Check sheet for the modelled part. Datum: model origin and axes. Units: mm. A direction names the side the tool comes from. Round coordinates to 2 decimals unless told otherwise and drop trailing zeros. One line per item, written item: value.
Autodesk Inventor part; units mm, degrees
ref_plane "YZ Plane" through (0, 0, 0) normal (1, 0, 0) x (0, 1, 0)
ref_plane "XZ Plane" through (0, 0, 0) normal (0, 1, 0) x (-1, 0, 0)
ref_plane "XY Plane" through (0, 0, 0) normal (0, 0, 1) x (1, 0, 0)
sketch "Sketch_1" plane through (0, 0, 0) normal (0, 0, 1) x (1, 0, 0)
  arc A0 (-7.5, 2) -> (-7.2, 1.7) centre (-7.2, 2) ccw
  line L0 (-7.2, 1.7) -> (-6.4, 1.7)
  line L1 (-6.4, 1.7) -> (-6.4, 2.85)
  line L2 (-6.4, 2.85) -> (-3.8, 2.85)
  line L3 (-3.8, 2.85) -> (-2.8, 1.85)
  line L4 (-2.8, 1.85) -> (-2.8, 0.5196)
  line L5 (-2.8, 0.5196) -> (-2.5, 0)
  line L6 (-2.5, 0) -> (-2.8, -0.5196)
  line L7 (-2.8, -0.5196) -> (-2.8, -1.85)
  line L8 (-2.8, -1.85) -> (-3.8, -2.85)
  line L9 (-3.8, -2.85) -> (-6.4, -2.85)
  line L10 (-6.4, -2.85) -> (-6.4, -1.7)
  line L11 (-6.4, -1.7) -> (-7.2, -1.7)
  arc A1 (-7.2, -1.7) -> (-7.5, -2) centre (-7.2, -2) ccw
  line L12 (-7.5, -2) -> (-7.5, -6.5)
  arc A2 (-7.5, -6.5) -> (-6.5, -7.5) centre (-6.5, -6.5) ccw
  line L13 (-6.5, -7.5) -> (-2, -7.5)
  arc A3 (-2, -7.5) -> (-1.7, -7.2) centre (-2, -7.2) ccw
  line L14 (-1.7, -7.2) -> (-1.7, -6.4)
  line L15 (-1.7, -6.4) -> (-2.85, -6.4)
  line L16 (-2.85, -6.4) -> (-2.85, -3.8)
  line L17 (-2.85, -3.8) -> (-1.85, -2.8)
  line L18 (-1.85, -2.8) -> (-0.5196, -2.8)
  line L19 (-0.5196, -2.8) -> (0, -2.5)
  line L20 (0, -2.5) -> (0.5196, -2.8)
  line L21 (0.5196, -2.8) -> (1.85, -2.8)
  line L22 (1.85, -2.8) -> (2.85, -3.8)
  line L23 (2.85, -3.8) -> (2.85, -6.4)
  line L24 (2.85, -6.4) -> (1.7, -6.4)
  line L25 (1.7, -6.4) -> (1.7, -7.2)
  arc A4 (1.7, -7.2) -> (2, -7.5) centre (2, -7.2) ccw
  line L26 (2, -7.5) -> (6.5, -7.5)
  arc A5 (6.5, -7.5) -> (7.5, -6.5) centre (6.5, -6.5) ccw
  line L27 (7.5, -6.5) -> (7.5, -2)
  arc A6 (7.5, -2) -> (7.2, -1.7) centre (7.2, -2) ccw
  line L28 (7.2, -1.7) -> (6.4, -1.7)
  line L29 (6.4, -1.7) -> (6.4, -2.85)
  line L30 (6.4, -2.85) -> (3.8, -2.85)
  line L31 (3.8, -2.85) -> (2.8, -1.85)
  line L32 (2.8, -1.85) -> (2.8, -0.5196)
  line L33 (2.8, -0.5196) -> (2.5, 0)
  line L34 (2.5, 0) -> (2.8, 0.5196)
  line L35 (2.8, 0.5196) -> (2.8, 1.85)
  line L36 (2.8, 1.85) -> (3.8, 2.85)
  line L37 (3.8, 2.85) -> (6.4, 2.85)
  line L38 (6.4, 2.85) -> (6.4, 1.7)
  line L39 (6.4, 1.7) -> (7.2, 1.7)
  arc A7 (7.2, 1.7) -> (7.5, 2) centre (7.2, 2) ccw
  line L40 (7.5, 2) -> (7.5, 6.5)
  arc A8 (7.5, 6.5) -> (6.5, 7.5) centre (6.5, 6.5) ccw
  line L41 (6.5, 7.5) -> (2, 7.5)
  arc A9 (2, 7.5) -> (1.7, 7.2) centre (2, 7.2) ccw
  line L42 (1.7, 7.2) -> (1.7, 6.4)
  line L43 (1.7, 6.4) -> (2.85, 6.4)
  line L44 (2.85, 6.4) -> (2.85, 3.8)
  line L45 (2.85, 3.8) -> (1.85, 2.8)
  line L46 (1.85, 2.8) -> (0.5196, 2.8)
  line L47 (0.5196, 2.8) -> (0, 2.5)
  line L48 (0, 2.5) -> (-0.5196, 2.8)
  line L49 (-0.5196, 2.8) -> (-1.85, 2.8)
  line L50 (-1.85, 2.8) -> (-2.85, 3.8)
  line L51 (-2.85, 3.8) -> (-2.85, 6.4)
  line L52 (-2.85, 6.4) -> (-1.7, 6.4)
  line L53 (-1.7, 6.4) -> (-1.7, 7.2)
  arc A10 (-1.7, 7.2) -> (-2, 7.5) centre (-2, 7.2) ccw
  line L54 (-2, 7.5) -> (-6.5, 7.5)
  arc A11 (-6.5, 7.5) -> (-7.5, 6.5) centre (-6.5, 6.5) ccw
  line L55 (-7.5, 6.5) -> (-7.5, 2)
  circle A12 centre (0, 0) radius 1.25
extrude "Extrusion1" add sketch "Sketch_1" along normal blind 120
equation "\"d0\" = L"
equation "\"L\" = 120"
properties part number "HFS3-1515-120"
Q1. Access from +Z, -Z, +X, -X, +Y, -Y to the whole of each face (thin tool, end or side, straight path). Record for faces 4 (the flat face through (7.5, -4, 59)), 5 (the flat face through (2.85, 5, 59)).
Completed:
face 4: +Z, -Z, +X, +Y, -Y
face 5: +Z, -Z
Q2. Scan lines: line 1 (X direction, y = 6, z = 17.5); line 2 (Y direction, x = 0, z = 49.5). Record each from-to range of solid material in increasing order. Write a range as [from, to].
Completed:
line 1: [-7.5, -2.85], [2.85, 7.5]
line 2: [-2.5, -1.25], [1.25, 2.5]
Q3. Depth check by flat-ended pin: P1, Ø0.9, axis at y = -7, z = 89.5, coming from the +X side; P2, Ø1.5, axis at x = -0.5, z = 35.5, coming from the -Y side; P3, Ø0.7, axis at x = -1.5, z = 31.5, coming from the -Y side. Enter the tip coordinate at first touch or a pass-through.
Completed:
P1: x = 7.5
P2: y = -2.8
P3: y = -7.46
Q4. Draft check along X on faces 1 (the flat face through (0, 2, 0)), 2 (the cylindrical face through (-0.27, 1.22, 59.16)), 3 (the flat face through (-7.5, -4, 59)). Enter one of: pulls with the +X half, pulls with the -X half, needs draft (parallel to the pull), parting line crosses it, or undercut.
Completed:
face 1: needs draft
face 2: undercut
face 3: pulls with the -X half
